Input: part model. Units: mm. Frame: model coordinates. Give positions to 0.01 mm unless a question says otherwise; leave off trailing zeros. Loops run counter-clockwise (first coordinate to the right, second up) from the corner with the lowest first, then second, coordinate; pieces in that order, holes last. Notation, with made-up numbers: (20.25, 49) -> (68.25, 49) arc R16 ccw to (68.25, 59) -> close; hole circle Ø2 at (61, 37.5). An arc over 180 degrees is marked (long way). Use CSV: the item, a comma, the result in double quotes.
```python
from build123d import *

# Parameters (mm, degrees)
SKETCH1_R           = 76.182
SKETCH1_R_2         = 49.3
BOSS_EXTRUDE1_DEPTH = 2.5
SKETCH2_R           = 1.6
CUT_EXTRUDE1_DEPTH  = 108.766619359
SKETCH3_R           = 2.2
CUT_EXTRUDE2_DEPTH  = 108.766619359
CIRPATTERN1_COUNT   = 9


with BuildPart() as part:
    # Sketch1 → Boss-Extrude1 (new body)
    with BuildSketch(Plane(origin=(0, 0, 0), x_dir=(1, 0, 0), z_dir=(0, 1, 0))):
        with Locations(Location((0, 0, 0), (0, 0, 270))):
            Circle(SKETCH1_R)
        with Locations(Location((0, 0, 0), (0, 0, 270))):
            Circle(SKETCH1_R_2, mode=Mode.SUBTRACT)
    extrude(amount=BOSS_EXTRUDE1_DEPTH)

    # Sketch2 → Cut-Extrude1 (cut, through all)
    with BuildSketch(Plane(origin=(0, 2.5, 0), x_dir=(1, 0, 0), z_dir=(0, 1, 0))):
        with Locations(Location((-65.748850074, -5.752279021, 0), (0, 0, 270))):
            Circle(SKETCH2_R)
    cut_extrude1 = extrude(amount=-CUT_EXTRUDE1_DEPTH, mode=Mode.SUBTRACT)

    # Sketch3 → Cut-Extrude2 (cut, through all)
    with BuildSketch(Plane(origin=(0, 2.5, 0), x_dir=(1, 0, 0), z_dir=(0, 1, 0))):
        with Locations(Location((0, 59.18, 0), (0, 0, 270))):
            Circle(SKETCH3_R)
        with Locations(Location((29.59, 51.251383396, 0), (0, 0, 270))):
            Circle(SKETCH3_R)
        with Locations(Location((51.251383396, 29.59, 0), (0, 0, 270))):
            Circle(SKETCH3_R)
        with Locations(Location((59.18, 0, 0), (0, 0, 270))):
            Circle(SKETCH3_R)
        with Locations(Location((51.251383396, -29.59, 0), (0, 0, 270))):
            Circle(SKETCH3_R)
        with Locations(Location((29.59, -51.251383396, 0), (0, 0, 270))):
            Circle(SKETCH3_R)
        with Locations(Location((0, -59.18, 0), (0, 0, 270))):
            Circle(SKETCH3_R)
        with Locations(Location((-29.59, -51.251383396, 0), (0, 0, 270))):
            Circle(SKETCH3_R)
        with Locations(Location((-51.251383396, -29.59, 0), (0, 0, 270))):
            Circle(SKETCH3_R)
        with Locations(Location((-59.18, 0, 0), (0, 0, 270))):
            Circle(SKETCH3_R)
        with Locations(Location((-51.251383396, 29.59, 0), (0, 0, 270))):
            Circle(SKETCH3_R)
        with Locations(Location((-29.59, 51.251383396, 0), (0, 0, 270))):
            Circle(SKETCH3_R)
    extrude(amount=-CUT_EXTRUDE2_DEPTH, mode=Mode.SUBTRACT)

    # CirPattern1: Cut-Extrude1 ×9 about axis
    cirpattern1_axis = Axis((0, 0, 0), (0, 1, 0))
    for i in range(1, CIRPATTERN1_COUNT):
        add(cut_extrude1.rotate(cirpattern1_axis, i * 360 / CIRPATTERN1_COUNT), mode=Mode.SUBTRACT)


solid = part.part
```
1) Section query C-C (z = 59.18). Return loops of the section in (x, y).
From the geometry:
outline,"(-47.97, 0) -> (-2.2, 0) -> (-2.2, 2.5) -> (-47.97, 2.5) -> close; (2.2, 0) -> (47.97, 0) -> (47.97, 2.5) -> (2.2, 2.5) -> close"
2) Contact query for flat-ended pins moving along their axis: pin 1 (1.5 mm diameter, centred on x = 49, y = 0.5, fed in from +Z); pin 2 (1.5 mm diameter, centred on x = -53.5, y = 1, fed in from -Z). Output: stop coordinate, or through.
From the geometry:
pin 1,"stops at z = 58.95"
pin 2,"stops at z = -54.96"
3) Mould query, pull axis X, two halves, no side actions, for faces 1 (the flat face through (-50, 0, -1)), 2 (the cylindrical face through (22.883, 1.232, 72.664)), 3 (the cylindrical face through (-1.339, 1.268, -60.926)), 4 (the cylindrical face through (0.097, 1.268, 56.982)). Classes: pulls with the +X half, pulls with the -X half, needs draft (parallel to the pull), parting line crosses it, or undercut.
From the geometry:
face 1,"needs draft"
face 2,"parting line crosses it"
face 3,"undercut"
face 4,"undercut"
4) Ray query, line 1 (X direction, y = 1.2, z = 0); line 2 (X direction, y = 0.75, z = -59.18); line 3 (Z direction, x = -7, y = 0.3). Return the intervals inside material, ascending.
From the geometry:
line 1,"x = -76.18 to -61.38, -56.98 to -49.3, 49.3 to 56.98, 61.38 to 76.18"
line 2,"x = -47.97 to -2.2, 2.2 to 26.42, 29.36 to 47.97"
line 3,"z = -75.86 to -48.8, 48.8 to 64.75, 66.75 to 75.86"
5) Section query B-B (x = -22.5). Return loops of the section in (y, z).
From the geometry:
outline,"(0, -72.78) -> (2.5, -72.78) -> (2.5, -43.87) -> (0, -43.87) -> close; (0, 43.87) -> (2.5, 43.87) -> (2.5, 72.78) -> (0, 72.78) -> close"
6) Section query A-A (z = 0). Return loops of the section in (x, y).
From the geometry:
outline,"(-76.18, 0) -> (-61.38, 0) -> (-61.38, 2.5) -> (-76.18, 2.5) -> close; (-56.98, 0) -> (-49.3, 0) -> (-49.3, 2.5) -> (-56.98, 2.5) -> close; (49.3, 0) -> (56.98, 0) -> (56.98, 2.5) -> (49.3, 2.5) -> close; (61.38, 0) -> (76.18, 0) -> (76.18, 2.5) -> (61.38, 2.5) -> close"
7) Section query D-D (y = 0.55). Give the number of separate pieces and of enclosed holes in the cut face, then the cut area to 3 significant figures.
From the geometry:
separate pieces,"1"
enclosed holes,"22"
area,"10,300 mm^2"
